Job drawing, mm, ordinate dimensions from the low corner. One solid piece. A direction names the side the tool comes from. Coordinates: 2 decimals unless noted, no trailing zeros. Order: outer loops, then holes, each group sorted by start corner. A loop starts at its lowest first (then second) coordinate and runs counter-clockwise, first axis right, second up. Notation, with made-up numbers: M 29,76 L 69,76 A19 ccw 69,84 Z; hole C -6,0.5 d6. An arc over 180 degrees is marked long. Write item = value, one per line.
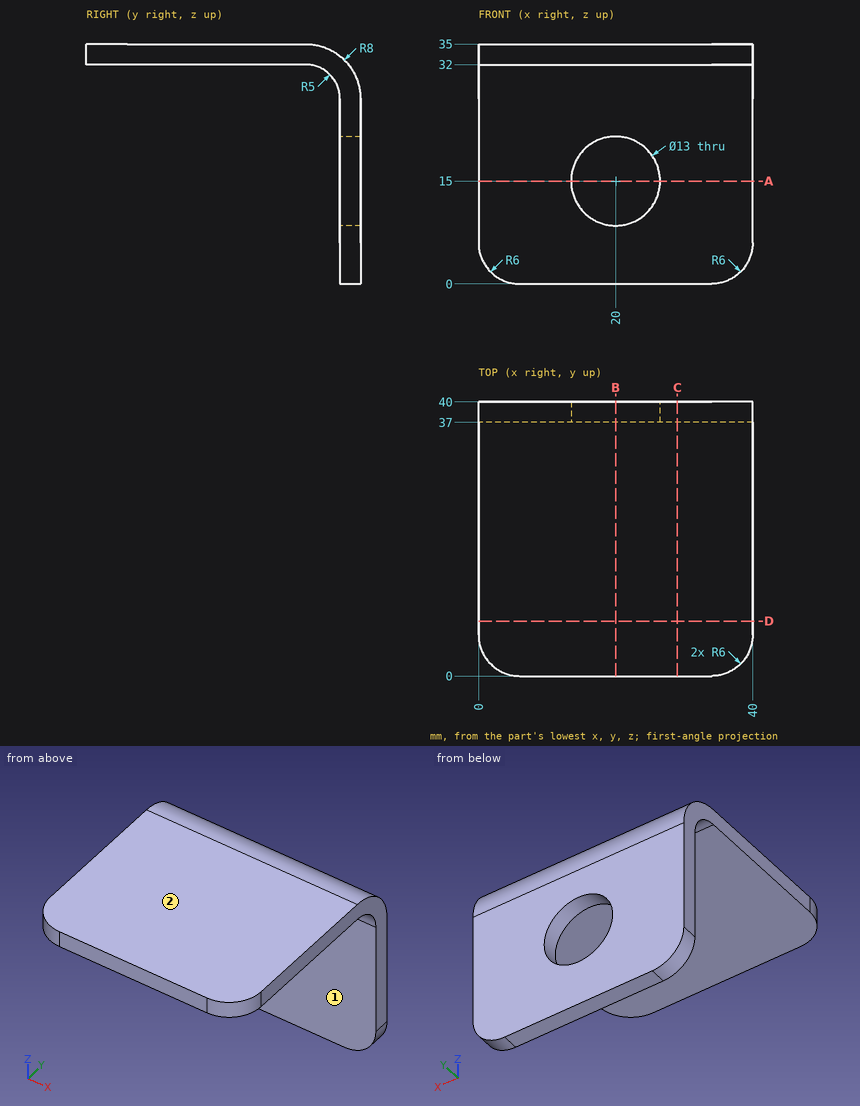
(1) Tool access for the marked faces 1 and 2: list every direction of +Z, -Z, +X, -X, +Y, -Y with a clear straight run to the whole face (end or side of a thin tool).
Evaluation:
face_1 = -Z, +X, -X, -Y
face_2 = +Z, +X, -X, +Y, -Y
(2) Slice it at D-D, the plane y = 8. Write the cut outline in (x, z), then the cut area to 3 significant figures.
Evaluation:
outline = M 0,32 L 40,32 L 40,35 L 0,35 Z
area = 120 mm²
(3) Slice it at C-C, the plane x = 29. Write the cut outline in (y, z).
Evaluation:
outline = M 0,32 L 32,32 A5 cw 37,27 L 37,0 L 40,0 L 40,27 A8 ccw 32,35 L 0,35 Z
(4) Pin check, flat tips, straight feed: pin 1 Ø8 at (x, z) = (6, 29) entering from +Y; pin 2 Ø16 at (x, y) = (20.5, 12) entering from -Z; pin 3 Ø12 at (y, z) = (28.5, 18) entering from +X. Stop position of each tip, or through.
Evaluation:
pin_1 = 40
pin_2 = 32
pin_3 = through
(5) Slice it at B-B, the plane x = 20. Write the cut outline in (y, z), then the cut area to 3 significant figures.
Evaluation:
outline = M 0,32 L 32,32 A5 cw 37,27 L 37,21.5 L 40,21.5 L 40,27 A8 ccw 32,35 L 0,35 Z; M 37,0 L 40,0 L 40,8.5 L 37,8.5 Z
area = 169 mm²
(6) Slice it at A-A, the plane z = 15. Write the cut outline in (x, y), then the cut area to 3 significant figures.
Evaluation:
outline = M 0,37 L 13.5,37 L 13.5,40 L 0,40 Z; M 26.5,37 L 40,37 L 40,40 L 26.5,40 Z
area = 81.0 mm²
(7) Wall check: line 1 (Z direction, x = 19.5, y = 15); line 2 (Y direction, x = 35, z = 13.5); line 3 (Z direction, x = 20, y = 38.2). Give the ranges that are in metal, low to high. Write a range as from..to.
Evaluation:
line_1 = 32..35
line_2 = 37..40
line_3 = 0..8.5, 21.5..32.06
